Autodesk Inventor part; units mm, degrees
ref_plane "YZ Plane" through (0, 0, 0) normal (1, 0, 0) x (0, 1, 0)
ref_plane "XZ Plane" through (0, 0, 0) normal (0, 1, 0) x (-1, 0, 0)
ref_plane "XY Plane" through (0, 0, 0) normal (0, 0, 1) x (1, 0, 0)
sketch "Sketch1" plane through (0, 0, 0) normal (0, 0, 1) x (1, 0, 0)
  line L0 (0.1713, 1.5278) -> (0.1713, -1.4722)
  line L1 (0.1713, 1.5278) -> (0.1713, 6.5278)
  line L2 (0.1713, -1.4722) -> (0.1713, -6.4722)
  line L3 (0.1713, -6.4722) -> (146.8575, -6.4722)
  line L4 (152.2423, 6.5278) -> (0.1713, 6.5278)
  line L5 (146.8575, -6.4722) -> (254.1159, -113.7306)
  line L6 (263.3083, -104.5382) -> (152.2423, 6.5278)
  line L7 (254.1159, -113.7306) -> (263.3083, -104.5382)
  line L8 (40.1713, -6.4722) -> (40.1713, -4.4722)
  line L9 (232.9494, -32.7504) -> (212.235, -53.4648)
  circle A0 centre (225.1713, -24.9722) radius 8.5
  circle A1 centre (225.1713, -24.9722) radius 11
  line L10 (217.3931, -17.194) -> (196.6786, -37.9085)
  line L11 (182.9494, -82.7504) -> (203.0426, -62.6572)
  line L12 (167.3931, -67.194) -> (187.4862, -47.1009)
  circle A2 centre (175.1713, -74.9722) radius 8.5
  circle A3 centre (175.1713, -74.9722) radius 11
  line L13 (86.1713, -24.9722) -> (86.1713, -6.4722)
  line L14 (64.1713, -24.9722) -> (64.1713, -6.4722)
  circle A4 centre (75.1713, -24.9722) radius 8.5
  circle A5 centre (75.1713, -24.9722) radius 11
  line L15 (86.1713, 25.0278) -> (86.1713, 6.5278)
  circle A6 centre (75.1713, 25.0278) radius 8.5
  circle A7 centre (75.1713, 25.0278) radius 11
  line L16 (64.1713, 25.0278) -> (64.1713, 6.5278)
  line L17 (40.1713, 4.5278) -> (40.1713, 6.5278)
  line L18 (40.1713, 4.5278) -> (151.4139, 4.5278)
  line L19 (151.4139, 4.5278) -> (260.4799, -104.5382)
  line L20 (260.4799, -104.5382) -> (254.1159, -110.9022)
  line L21 (254.1159, -110.9022) -> (147.686, -4.4722)
  line L22 (147.686, -4.4722) -> (40.1713, -4.4722)
  point P0 (0, 0)
  point P1 (0.1713, 0.0278)
  point P2 (0.1713, 0.0278)
  point P3 (0.1713, -3.9722)
  point P4 (40.1713, -3.9722)
  point P5 (76.2068, 6.5278)
  point P6 (86.1713, 6.5278)
  point P7 (64.1713, 6.5278)
  point P8 (86.1713, -6.4722)
  point P9 (64.1713, -6.4722)
  point P10 (203.0426, -62.6572)
  point P11 (187.4862, -47.1009)
  point P12 (196.6786, -37.9085)
  point P13 (212.235, -53.4648)
extrude "Extrusion4" add sketch "Sketch1" along normal blind 60 contours L4 L6 L7 L5 L3 L8 L22 L21 L20 L19 L18 L17
extrude "Extrusion5" add sketch "Sketch1" along normal blind 10 contours L1 L4 L17 L18 L19 L20 L21 L22 L8 L3 L2 L0 | L16 A7 L15 L4 | L3 L13 A5 L14 | A7 | A5 | L10 A1 L9 L6 | L5 L11 A3 L12 | A1 | A3
properties part number "hold_right_sim"
Can you work these out from the model? Positions are in its coordinate system, mm. A direction names the side the tool comes from. Coordinates: 2 decimals unless noted, no trailing zeros. Loops run counter-clockwise (first coordinate to the right, second up) from the corner with the lowest first, then second, coordinate; pieces in that order, holes last. Notation, with made-up numbers: M 30,13 L 43,13 A30 cw 43,41 Z; hole C -23.75,-33.75 d7. An arc over 180 degrees is marked long. Answer as CSV lines item,"result". Start each with the question number.
1. Thinking about a two-plate mould opening in X: for faces 1 (the face through (74.929, 36.025, 4.93)), 2 (the face through (232.777, -17.025, 4.93)), 3 (the face through (64.171, 16, 5)), which applies, +X half, -X half, draft (parallel to the pull), parting line (faces both ways), or undercut?
2. Suppose I cut it at B-B, the plane z = 40.5. List the corners of the cut face in (x, y) for me, plus the area to 3 significant figures.
3. If I drill on probe 1 along Y at (x, z) = (78, 41); probe 2 along Y at (x, z) = (151, 23.5); probe 3 along X at (y, z) = (-94.5, 13.5), over which ranges is the centre line in solid material (lowest first)? Write a range as [from, to].
4. Suppose I cut it at D-D, the plane y = -72. List the corners of the cut face in (x, z) for me, plus the area to 3 significant figures.
5. For faces 4 (the face through (75, -14, 10)), 5 (the face through (86.171, -16, 5)), 6 (the face through (207.181, -27.406, 4.93)), 7 (the face through (205.18, -49.24, 34.65)), which set-ups out of +Z, -Z, +X, -X, +Y, -Y let a thin tool reach every point of the face, with its end or its side?
6. For pin 1 Ø1.6 at (y, z) = (-6, 33) entering from -X; pin 2 Ø12 at (y, z) = (-25, 21.5) entering from -X; pin 3 Ø22 at (x, y) = (75.17, -24.97) entering from +Z, each with a flat end and sliding along its axis, tell me the tip position at first contact or that it passes through.
7. Suppose I cut it at C-C, the plane y = -21.5. List the corners of the cut face in (x, z) for me, plus the area to 3 significant figures.
8. Suppose I cut it at A-A, the plane x = 175. List the corners of the cut face in (y, z) for me, plus the area to 3 significant figures.
Output:
1,face 1,"parting line"
1,face 2,"undercut"
1,face 3,"-X half"
2,outline,"M 40.17,-6.47 L 146.86,-6.47 L 254.12,-113.73 L 263.31,-104.54 L 152.24,6.53 L 40.17,6.53 L 40.17,4.53 L 151.41,4.53 L 260.48,-104.54 L 254.12,-110.9 L 147.69,-4.47 L 40.17,-4.47 Z"
2,area,"1,070 mm^2"
3,probe 1,"y = [-6.47, -4.47], [4.53, 6.53]"
3,probe 2,"y = [-10.61, -7.79], [4.53, 6.53]"
3,probe 3,"x = [234.89, 237.71], [250.44, 253.27]"
4,outline,"M 164.58,0 L 167.21,0 L 167.21,10 L 164.58,10 Z; M 183.13,0 L 193.7,0 L 193.7,10 L 183.13,10 Z; M 212.39,0 L 230.77,0 L 230.77,60 L 227.94,60 L 227.94,10 L 215.21,10 L 215.21,60 L 212.39,60 Z"
4,area,"599 mm^2"
5,face 4,"+Z, -X, -Y"
5,face 5,"+Z, -Z, -Y"
5,face 6,"+Z, -Z, +Y"
5,face 7,"+Z"
6,pin 1,"stops at x = 40.17"
6,pin 2,"stops at x = 159.39"
6,pin 3,"stops at z = 10"
7,outline,"M 64.17,0 L 67.41,0 L 67.41,10 L 64.17,10 Z; M 82.93,0 L 86.17,0 L 86.17,10 L 82.93,10 Z; M 161.89,0 L 180.27,0 L 180.27,60 L 177.44,60 L 177.44,10 L 164.71,10 L 164.71,60 L 161.89,60 Z; M 213.09,0 L 217.41,0 L 217.41,10 L 213.09,10 Z; M 232.93,0 L 235.61,0 L 235.61,10 L 232.93,10 Z"
7,area,"602 mm^2"
8,outline,"M -85.97,0 L -83.47,0 L -83.47,10 L -85.97,10 Z; M -66.47,0 L -59.59,0 L -59.59,10 L -66.47,10 Z; M -34.61,0 L -16.23,0 L -16.23,60 L -19.06,60 L -19.06,10 L -31.79,10 L -31.79,60 L -34.61,60 Z"
8,area,"561 mm^2"
